```python
from build123d import *

# Parameters (mm, degrees)
SKETCH1_W               = 100
SKETCH1_H               = 100
BOSS_EXTRUDE1_DEPTH     = 26
SKETCH2_R               = 4.005
SKETCH2_R_2             = 4.5
CUT_EXTRUDE1_DEPTH      = 23
SKETCH4_R               = 7.55
CUT_EXTRUDE2_DEPTH      = 24
CUT_EXTRUDE3_DEPTH      = 76.339232807
CUT_EXTRUDE3_DEPTH_BACK = 76.339232807
SKETCH5_R               = 4.5
FILLET1_R               = 40


with BuildPart() as part:
    # Sketch1 → Boss-Extrude1 (new body)
    with BuildSketch(Plane.XY):
        Rectangle(SKETCH1_W, SKETCH1_H)
    extrude(amount=BOSS_EXTRUDE1_DEPTH)

    # Sketch2 → Cut-Extrude1 (cut)
    with BuildSketch(Plane.XY.offset(26)):
        with Locations((0, 28.499999998)):
            Circle(SKETCH2_R)
        with Locations((-26.5, -26.500000001)):
            Circle(SKETCH2_R)
        with Locations((26.5, -26.500000001)):
            Circle(SKETCH2_R)
        Circle(SKETCH2_R_2)
    extrude(amount=-CUT_EXTRUDE1_DEPTH, mode=Mode.SUBTRACT)

    # Sketch4 → Cut-Extrude2 (cut)
    with BuildSketch(Plane.XY.offset(26)):
        with Locations((-26.5, 28.499999998)):
            Circle(SKETCH4_R)
        with Locations((26.5, 28.499999998)):
            Circle(SKETCH4_R)
        with Locations((0, -26.500000002)):
            Circle(SKETCH4_R)
    extrude(amount=-CUT_EXTRUDE2_DEPTH, mode=Mode.SUBTRACT)

    # Sketch5 → Cut-Extrude3 (cut, two sides: drawn at the far end of the back side and taken through both)
    with BuildSketch(Plane.XY.offset(26).offset(-CUT_EXTRUDE3_DEPTH_BACK)):
        with Locations((-26.5, 28.499999998)):
            Circle(SKETCH5_R)
        with Locations((26.5, 28.499999998)):
            Circle(SKETCH5_R)
        with Locations((0, -26.500000002)):
            Circle(SKETCH5_R)
    extrude(amount=CUT_EXTRUDE3_DEPTH + CUT_EXTRUDE3_DEPTH_BACK, mode=Mode.SUBTRACT)

    # Fillet1
    fillet1_edges = [part.edges().sort_by_distance(p)[0] for p in [
        (50, -50, 13),
        (-50, -50, 13),
        (-50, 50, 13),
        (50, 50, 13),
    ]]
    fillet(fillet1_edges, radius=FILLET1_R)


solid = part.part
```
Can you work these out from the model? Positions are in its coordinate system, mm. A direction names the side the tool comes from. Coordinates: 2 decimals unless noted, no trailing zeros. Order: outer loops, then holes, each group sorted by start corner. A loop starts at its lowest first (then second) coordinate and runs counter-clockwise, first axis right, second up. Notation, with made-up numbers: (72, 30.5) - (89, 30.5) arc R25 cw to (89, 67.5) - close; hole circle Ø8 at (-9, -3). An arc over 180 degrees is marked (long way). Answer in a Markdown table with one row per item.
1. Suppose I cut it at A-A (z = 16). Please give me the cut outline in (x, y) (3 decimals).
Reply:
| item | result |
|---|---|
| outline | (-50, -10) arc R40 ccw to (-10, -50) - (10, -50) arc R40 ccw to (50, -10) - (50, 10) arc R40 ccw to (10, 50) - (-10, 50) arc R40 ccw to (-50, 10) - close; hole circle Ø15.1 at (-26.5, 28.5); hole circle Ø8.01 at (-26.5, -26.5); hole circle Ø15.1 at (0, -26.5); hole circle Ø9 at (0, 0); hole circle Ø8.01 at (0, 28.5); hole circle Ø15.1 at (26.5, 28.5); hole circle Ø8.01 at (26.5, -26.5) |
2. Suppose I cut it at C-C (y = -26.5). Please give me the cut outline in (x, z) (3 decimals).
Reply:
| item | result |
|---|---|
| outline | (-46.438, 0) - (-4.5, 0) - (-4.5, 2) - (-7.55, 2) - (-7.55, 26) - (-22.495, 26) - (-22.495, 3) - (-30.505, 3) - (-30.505, 26) - (-46.438, 26) - close; (4.5, 0) - (46.438, 0) - (46.438, 26) - (30.505, 26) - (30.505, 3) - (22.495, 3) - (22.495, 26) - (7.55, 26) - (7.55, 2) - (4.5, 2) - close |
3. Suppose I cut it at B-B (x = 0). Please give me the cut outline in (y, z) (3 decimals).
Reply:
| item | result |
|---|---|
| outline | (-50, 0) - (-31, 0) - (-31, 2) - (-34.05, 2) - (-34.05, 26) - (-50, 26) - close; (-22, 0) - (50, 0) - (50, 26) - (32.505, 26) - (32.505, 3) - (24.495, 3) - (24.495, 26) - (4.5, 26) - (4.5, 3) - (-4.5, 3) - (-4.5, 26) - (-18.95, 26) - (-18.95, 2) - (-22, 2) - close |
4. If we mould it in two halves opening along Y, with no side actions, what happens to faces 1 (the cylindrical face through (1.85, 24.95, 14.66)), 2 (the flat face through (-1, -10, 26)), 3 (the cylindrical face through (-29.678, -28.937, 14.661)), 4 (the flat face through (0, -50, 13))? For each: pulls with the +Y half, pulls with the -Y half, needs draft (parallel to the pull), parting line crosses it, or undercut.
Reply:
| item | result |
|---|---|
| face 1 | undercut |
| face 2 | needs draft |
| face 3 | undercut |
| face 4 | pulls with the -Y half |
5. For faces 5 (the cylindrical face through (25.517, 35.986, 14.168)), 6 (the flat face through (50, 0, 13)), which set-ups out of +Z, -Z, +X, -X, +Y, -Y let a thin tool reach every point of the face, with its end or its side?
Reply:
| item | result |
|---|---|
| face 5 | +Z |
| face 6 | +Z, -Z, +X, +Y, -Y |
6. Suppose I cut it at D-D (y = 42). Please give me the cut outline in (x, z), and give its area (3 significant figures).
Reply:
| item | result |
|---|---|
| outline | (-34, 0) - (34, 0) - (34, 26) - (-34, 26) - close |
| area | 1,770 mm^2 |
7. If I drill on line 1 along Y through (x, z) = (0, 13.75) (3 decimals); line 2 along Y through (x, z) = (0, 1.2); line 3 along X through (y, z) = (28.5, 13.25) (3 decimals), over which ranges is the centre line in solid material (lowest first)?
Reply:
| item | result |
|---|---|
| line 1 | y = -50 to -34.05, -18.95 to -4.5, 4.5 to 24.495, 32.505 to 50 |
| line 2 | y = -50 to -31, -22 to 50 |
| line 3 | x = -45.465 to -34.05, -18.95 to -4.005, 4.005 to 18.95, 34.05 to 45.465 |
8. For pin 1 (5 mm diameter, centred on y = 30.5, z = 16.5, fed in from -X); pin 2 (9 mm diameter, centred on x = -27.5, y = -26, fed in from +Z); pin 3 (3 mm diameter, centred on y = 18.5, z = 14, fed in from -X); pin 4 (12 mm diameter, centred on x = -26.5, y = 28.5, fed in from +Z), each with a flat end and sliding along its axis, tell me the tip position at first contact or that it passes through.
Reply:
| item | result |
|---|---|
| pin 1 | stops at x = -45.72 |
| pin 2 | stops at z = 26 |
| pin 3 | stops at x = -49.38 |
| pin 4 | stops at z = 2 |
